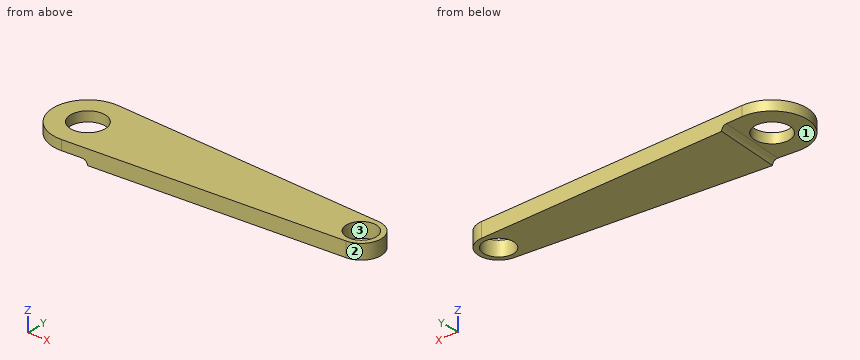
```python
from build123d import *

# Parameters (mm, degrees)
SKETCH1_R               = 88.9
SKETCH1_R_2             = 76.2
BOSS_EXTRUDE1_DEPTH     = 38.1
CUT_EXTRUDE1_DEPTH      = 940.915106169
CUT_EXTRUDE1_DEPTH_BACK = 940.915106169
SKETCH2_W               = 304.8
SKETCH2_H               = 25.4
FILLET1_R               = 25.4


with BuildPart() as part:
    # Sketch1 → Boss-Extrude1 (new, symmetric)
    with BuildSketch(Plane.XY):
        with BuildLine():
            Line((-688.801818182, 177.535307107), (704.041818182, 101.448746918))
            ThreePointArc((704.041818182, 101.448746918), (800.1, 0), (704.041818182, -101.448746918))
            Line((704.041818182, -101.448746918), (-688.801818182, -177.535307107))
            ThreePointArc((-688.801818182, -177.535307107), (-876.3, 0), (-688.801818182, 177.535307107))
        make_face()
        with Locations(Location((-698.5, 0, 0), (0, 0, 180))):
            Circle(SKETCH1_R, mode=Mode.SUBTRACT)
        with Locations(Location((698.5, 0, 0), (0, 0, 180))):
            Circle(SKETCH1_R_2, mode=Mode.SUBTRACT)
    extrude(amount=BOSS_EXTRUDE1_DEPTH, both=True)

    # Sketch2 → Cut-Extrude1 (cut, two sides: drawn at the far end of the back side and taken through both)
    with BuildSketch(Plane(origin=(7.62, -139.492027012, 0), x_dir=(0.998511288563344, 0.054545454545454695, 0), z_dir=(0.054545454545454695, -0.998511288563344, 0)).offset(-CUT_EXTRUDE1_DEPTH_BACK)):
        with Locations((-722.860135061, -25.4)):
            Rectangle(SKETCH2_W, SKETCH2_H)
    extrude(amount=CUT_EXTRUDE1_DEPTH + CUT_EXTRUDE1_DEPTH_BACK, mode=Mode.SUBTRACT)

    # Fillet1
    fillet1_edges = [part.edges().sort_by_distance(p)[0] for p in [
        (-571.338545978, 0.510632627, -12.7),
    ]]
    fillet(fillet1_edges, radius=FILLET1_R - 0.0001)  # a hair under: the kernel refuses the full size


solid = part.part
```
For this review, take the finished solid that the model builds, in its own axes (mm). Face numbers are marked on the shaded views. Give positions to 0.01 mm unless a question says otherwise; leave off trailing zeros. Order: outer loops, then holes, each group sorted by start corner. A loop starts at its lowest first (then second) coordinate and runs counter-clockwise, first axis right, second up.
1) Insertion check: pin 1 (10 mm diameter, centred on x = -664.5, z = 6.5, fed in from +Y); pin 2 (8 mm diameter, centred on y = -7, z = 22, fed in from +X); pin 3 (5 mm diameter, centred on x = -31.5, z = -16, fed in from +Y). Each pin has a flat end and moves straight along its axis. Give the tip position at first contact, or say it passes through.
2) Take a section at C-C (x = -368.5). Give the boundary of the cut face in (y, z), then the cut area to 3 significant figures.
3) The part is to be moulded in two halves that separate along Y. For the marked faces 1, 2 and 3, say which applies: released by +Y, released by -Y, zero draft, split by the parting line, or undercut.
4) Take a section at D-D (x = 540.5). Give the boundary of the cut face in (y, z).
5) Take a section at B-B (y = 40). State how many separate pieces and enclosed holes the cut face has, then the cut area to 3 significant figures.
6) Take a section at A-A (z = 25.5). Give the boundary of the cut face in (x, y).
7) Wall thickness on line 1 (Y direction, x = -698, z = 20); line 2 (X direction, y = 25, z = 9); line 3 (Y direction, x = 698.5, z = -7.5): over which ranges is each line inside the solid? List them lowest first.
Derived:
1. pin 1: stops at y = 176.48
1. pin 2: stops at x = 800.06
1. pin 3: stops at y = 141.77
2. outline: (-160.04, -38.1) - (160.04, -38.1) - (160.04, 38.1) - (-160.04, 38.1) - close
2. area: 24,400 mm2
3. face 1: zero draft
3. face 2: split by the parting line
3. face 3: undercut
4. outline: (-110.38, -38.1) - (110.38, -38.1) - (110.38, 38.1) - (-110.38, 38.1) - close
5. separate pieces: 3
5. enclosed holes: 0
5. area: 101,000 mm2
6. outline: (-688.8, -177.54) - (704.04, -101.45) arc R101.6 ccw to (704.04, 101.45) - (-688.8, 177.54) arc R177.8 ccw (long way) to start; hole circle Ø177.8 at (-698.5, 0); hole circle Ø152.4 at (698.5, 0)
7. line 1: y = -177.8 to -88.9, 88.9 to 177.8
7. line 2: x = -874.53 to -783.81, -613.19 to 626.52, 770.48 to 796.98
7. line 3: y = -101.75 to -76.2, 76.2 to 101.75
